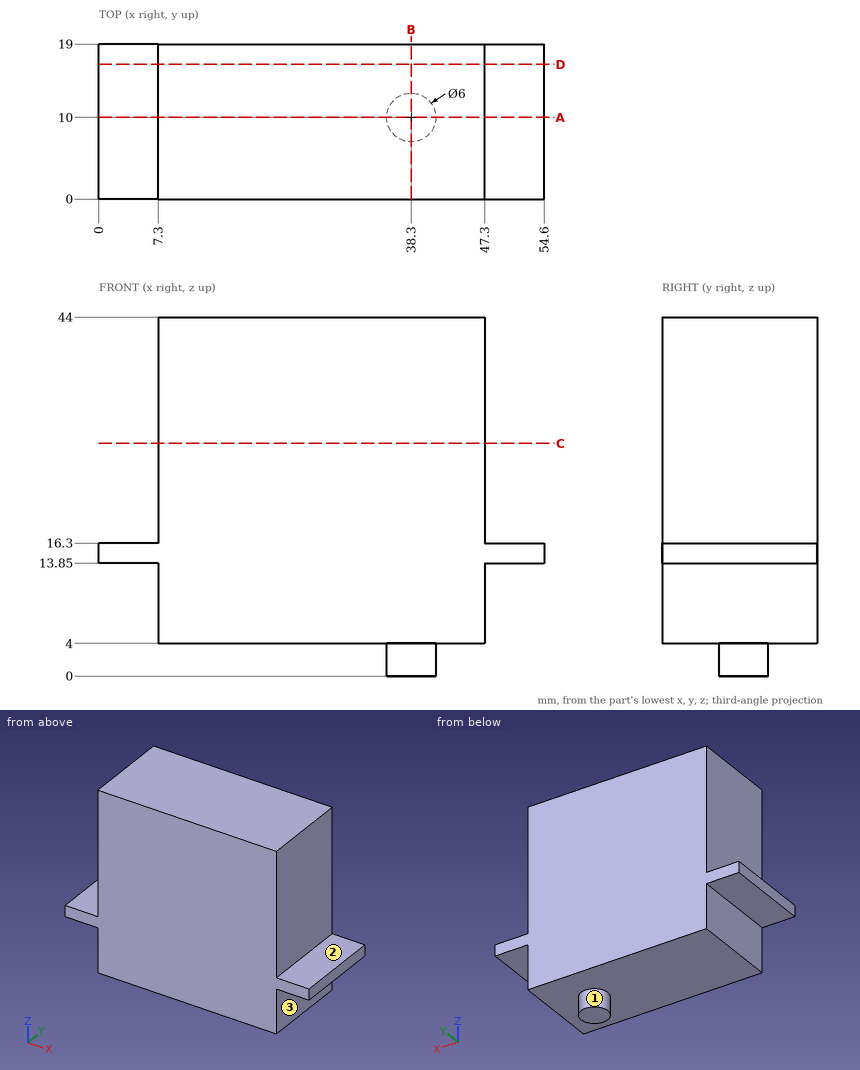
Input: dimensioned drawing with shaded views. Units: mm. Origin: part minimum x, y, z. A direction names the side the tool comes from. Give positions to 0.01 mm unless a question says otherwise; leave off trailing zeros. Write each loop counter-clockwise with the first axis right and the second up, starting at its lowest first coordinate (ties: lowest second). Pieces come first, ordered by that corner, then holes.
1. Section query B-B, the plane x = 38.3. Return loops of the section in (y, z), then the cut area to 3 significant figures.
2. Pin query (flat end, axial travel): P1, Ø9.5, axis at y = 7.5, z = 25, coming from the -X side; P2, Ø9.5, axis at y = 8.5, z = 31.5, coming from the +X side; P3, Ø6, axis at x = 52.5, y = 10, coming from the +Z side. Return the tip coordinate at first contact, or that it passes through.
3. Section query A-A, the plane y = 10. Return loops of the section in (x, z).
4. Section query D-D, the plane y = 16.5. Return loops of the section in (x, z).
5. Line query: probe 1 along X at (y, z) = (2.5, 19); probe 2 along Z at (x, y) = (29.5, 10); probe 3 along Z at (x, y) = (5, 12.75). Output: solid intervals per line, ascending.
6. Reachability of the marked faces 1, 2 and 3 from +Z, -Z, +X, -X, +Y, -Y: full face, straight path, thin tool, end or side. Return the list, or none.
7. Section query C-C, the plane z = 28.5. Return loops of the section in (x, y), then the cut area to 3 significant figures.
Computed:
1. outline: (0, 4) - (7, 4) - (7, 0) - (13, 0) - (13, 4) - (19, 4) - (19, 44) - (0, 44) - close
1. area: 784 mm2
2. P1: stops at x = 7.3
2. P2: stops at x = 47.3
2. P3: stops at z = 16.3
3. outline: (0, 13.85) - (7.3, 13.85) - (7.3, 4) - (35.3, 4) - (35.3, 0) - (41.3, 0) - (41.3, 4) - (47.3, 4) - (47.3, 13.85) - (54.6, 13.85) - (54.6, 16.3) - (47.3, 16.3) - (47.3, 44) - (7.3, 44) - (7.3, 16.3) - (0, 16.3) - close
4. outline: (0, 13.85) - (7.3, 13.85) - (7.3, 4) - (47.3, 4) - (47.3, 13.85) - (54.6, 13.85) - (54.6, 16.3) - (47.3, 16.3) - (47.3, 44) - (7.3, 44) - (7.3, 16.3) - (0, 16.3) - close
5. probe 1: x = 7.3 to 47.3
5. probe 2: z = 4 to 44
5. probe 3: z = 13.85 to 16.3
6. face 1: -Z
6. face 2: +Z, +X, +Y, -Y
6. face 3: -Z, +X, +Y, -Y
7. outline: (7.3, 0) - (47.3, 0) - (47.3, 19) - (7.3, 19) - close
7. area: 760 mm2
